Part model, mm, in its own coordinate system. A direction names the side the tool comes from. Give positions to 0.01 mm unless a question says otherwise; leave off trailing zeros. Loops run counter-clockwise (first coordinate to the right, second up) from the corner with the lowest first, then second, coordinate; pieces in that order, holes last. Notation, with made-up numbers: (-23.75, -13.5) -> (-3.75, -13.5) arc R34 ccw to (-3.75, 16.5) -> close; hole circle Ø2 at (0.5, 25). An arc over 180 degrees is marked (long way). Write item = value, one per line.
Autodesk Inventor part; units mm, degrees
ref_plane "Work Plane2" through (5.588, 0, 0) normal (1, 0, 0) x (0, 0, -1)
ref_plane "Work Plane3" through (5.588, 0, 0) normal (1, 0, 0) x (0, 0, -1)
ref_plane "Work Plane1" through (5.588, 0, 0) normal (1, 0, 0) x (0, 0, -1)
sketch "Sketch1" plane through (0, 0, 0) normal (1, 0, 0) x (0, 1, 0)
  circle A0 centre (0, 0) radius 23.368
  dimension "d0" = 46.736
extrude "Extrusion1" add sketch "Sketch1" along normal blind 5.588
ref_plane "Work Plane2" through (5.588, 0, 0) normal (1, 0, 0) x (0, 0, -1)
sketch "Sketch3" plane through (5.588, 0, 0) normal (1, 0, 0) x (0, 0, -1)
  line L0 (0, -3.4925) -> (0, 3.4925) construction
  line L1 (2.413, -3.4925) -> (2.413, 3.4925)
  line L2 (-2.413, 3.4925) -> (-2.413, -3.4925)
  arc A0 (-2.413, -3.4925) -> (2.413, -3.4925) centre (0, -3.4925) ccw
  arc A1 (2.413, 3.4925) -> (-2.413, 3.4925) centre (0, 3.4925) ccw
  point P0 (0, 0)
  dimension "d8" = 3.4925
  dimension "d9" = 4.826
extrude "Extrusion2" cut sketch "Sketch3" against normal blind 5.08
ref_plane "Work Plane3" through (5.588, 0, 0) normal (1, 0, 0) x (0, 0, -1)
sketch "Sketch6" plane through (5.588, 0, 0) normal (1, 0, 0) x (0, 0, -1)
  line L0 (0, 0) -> (0, 13.97)
  circle A0 centre (0, 13.97) radius 1.905
  circle A1 centre (-8.2114, 11.302) radius 1.905
  circle A2 centre (-13.2863, 4.317) radius 1.905
  circle A3 centre (-13.2863, -4.317) radius 1.905
  circle A4 centre (-8.2114, -11.302) radius 1.905
  circle A5 centre (0, -13.97) radius 1.905
  circle A6 centre (8.2114, -11.302) radius 1.905
  circle A7 centre (13.2863, -4.317) radius 1.905
  circle A8 centre (13.2863, 4.317) radius 1.905
  circle A9 centre (8.2114, 11.302) radius 1.905
  dimension "d16" = 13.97
  dimension "d17" = 3.81
  dimension "d20" = 360
extrude "Extrusion3" cut sketch "Sketch6" against normal blind 25.4
ref_plane "Work Plane1" through (5.588, 0, 0) normal (1, 0, 0) x (0, 0, -1)
sketch "Sketch7" plane through (5.588, 0, 0) normal (1, 0, 0) x (0, 0, -1)
  line L0 (0, 0) -> (0, -23.749) construction
  circle A0 centre (0, 0) radius 23.749
  dimension "d24" = 23.749
sketch "Sketch8" plane through (0, 0, 0) normal (0, 1, 0) x (-1, 0, 0)
  line L0 (0, -23.368) -> (0, 23.368)
  line L1 (0, -23.368) -> (0, -24.003)
  line L2 (0, -24.003) -> (-0.635, -24.003)
  line L3 (-0.635, -24.003) -> (-0.635, -23.368)
  line L4 (-0.635, -23.368) -> (0, -23.368)
  line L5 (0, -23.368) -> (-5.588, -23.368)
  line L6 (-0.635, -23.368) -> (0, -23.368)
  line L7 (-5.588, -23.368) -> (-5.588, -24.003)
  line L8 (-5.588, -24.003) -> (-4.953, -24.003)
  line L9 (-4.953, -24.003) -> (-4.953, -23.368)
  line L10 (-4.953, -23.368) -> (-5.588, -23.368)
  line L11 (0, 0) -> (-5.8379, 0)
  dimension "d25" = 0.635
  dimension "d26" = 0.635
  dimension "d27" = 0.635
  dimension "d28" = 0.635
revolve "Revolution2" add sketch "Sketch8" angle 360 about axis through (0, 0, 0) along (1, 0, 0)
properties part number "msheehan_wheel_small"
1) Slice it at B-B, the plane z = 0. List the corners of the cut face in (x, y) (1 decimal), and give its area (3 significant figures).
Resolved:
outline = (0, -24) -> (0.6, -24) -> (0.6, -23.4) -> (5, -23.4) -> (5, -24) -> (5.6, -24) -> (5.6, -15.9) -> (0, -15.9) -> close; (0, -12.1) -> (5.6, -12.1) -> (5.6, -5.9) -> (0.5, -5.9) -> (0.5, 5.9) -> (5.6, 5.9) -> (5.6, 12.1) -> (0, 12.1) -> close; (0, 15.9) -> (5.6, 15.9) -> (5.6, 24) -> (5, 24) -> (5, 23.4) -> (0.6, 23.4) -> (0.6, 24) -> (0, 24) -> close
area = 160 mm²
2) Pull direction Z, two halves, no side cores. Call faces 4 (the face through (3.084, -5.905, 0.053)), 5 (the face through (5.266, 23.432, 5.203)), 6 (the face through (4.953, -23, -5)): pulls with the +Z half, pulls with the -Z half, needs draft (parallel to the pull), parting line crosses it, or undercut.
Resolved:
face_4 = undercut
face_5 = parting line crosses it
face_6 = needs draft
3) Slice it at A-A, the plane y = 0. List the corners of the cut face in (x, z) (3 decimals), and give its area (3 significant figures).
Resolved:
outline = (0, -24.003) -> (0.635, -24.003) -> (0.635, -23.368) -> (4.953, -23.368) -> (4.953, -24.003) -> (5.588, -24.003) -> (5.588, -2.413) -> (0.508, -2.413) -> (0.508, 2.413) -> (5.588, 2.413) -> (5.588, 24.003) -> (4.953, 24.003) -> (4.953, 23.368) -> (0.635, 23.368) -> (0.635, 24.003) -> (0, 24.003) -> close
area = 238 mm²
4) Which spindle directions (+Z, -Z, +X, -X, +Y, -Y) get a long thin tool onto all of the face, cutting with end or side? Do faces 1 (the face through (0.635, -23, -5)), 2 (the face through (3.084, 5.905, -0.053)), 3 (the face through (2.83, -9.7, -9.24)). Say none if no direction does.
Resolved:
face_1 = none
face_2 = +X
face_3 = +X, -X
5) Slice it at C-C, the plane x = 4.35. Count the separate pieces of the cut face and the enclosed holes in it, and give its area (3 significant figures).
Resolved:
separate_pieces = 1
enclosed_holes = 11
area = 1,550 mm²
6) Slice it at D-D, the plane y = 13.97. List the corners of the cut face in (x, z) (3 decimals).
Resolved:
outline = (0, -19.519) -> (0.635, -19.519) -> (0.635, -18.732) -> (4.953, -18.732) -> (4.953, -19.519) -> (5.588, -19.519) -> (5.588, -1.905) -> (0, -1.905) -> close; (0, 1.905) -> (5.588, 1.905) -> (5.588, 19.519) -> (4.953, 19.519) -> (4.953, 18.732) -> (0.635, 18.732) -> (0.635, 19.519) -> (0, 19.519) -> close
7) Drop flat-ended pins along their axis: P1, Ø3, axis at x = 0.5, y = -10.5, coming from the +Z side; P2, Ø8, axis at y = -8.5, z = 7.5, coming from the -X side; P3, Ø2.5, axis at y = -11.3, z = 8.21, coming from the +X side; P4, Ø1.5, axis at x = 4, y = -1.5, coming from the +Z side. Give the stop position or say it passes through.
Resolved:
P1 = 22.25
P2 = 0
P3 = through
P4 = 23.36
8) Drill centre lines: line 1 along Y through (x, z) = (2.55, 0) (1 decimal); line 2 along Z through (x, y) = (2.7, 13) (3 decimals); line 3 along Z through (x, y) = (1.1, -11). Where is each one in solid material? Low to high. Write a range as [from, to].
Resolved:
line_1 = [-23.4, -15.9], [-12.1, -5.9], [5.9, 12.1], [15.9, 23.4]
line_2 = [-19.418, -9.075], [-7.348, -1.64], [1.64, 7.348], [9.075, 19.418]
line_3 = [-20.62, -10.09], [-6.33, 6.33], [10.09, 20.62]
